For this review, use the dimensioned drawing (mm, ordinates from the lowest corner) and the shaded views. Coordinates: 2 decimals unless noted, no trailing zeros. Loops run counter-clockwise (first coordinate to the right, second up) from the corner with the lowest first, then second, coordinate; pieces in that order, holes last. Notation, with made-up numbers: M 2.25,53.25 L 6.25,53.25 A16 ccw 6.25,62.25 Z; hole C -26,9 d6. An arc over 180 degrees is marked long. Write item = value, one per line. Start each with the question number.
Q1. Mouldability with a two-part tool opening along X and no side actions: class the marked faces 1 and 2 as released by +X, released by -X, zero draft, split by the parting line, or undercut.
Q2. We need section A-A on z = 15.24. Give the boundary of the cut face in (x, y).
Q3. We need section B-B on x = 15.24. Give the boundary of the cut face in (y, z), and give its area (3 significant figures).
Q4. We need section D-D on y = 24. Give the boundary of the cut face in (x, z).
Q5. Wall thickness on probe 1 along X at (y, z) = (35.7, 15.24); probe 2 along X at (y, z) = (23.5, 15.24): over which ranges is each line inside the solid? List them lowest first.
Q6. Clearance check with flat-ended pins moving along their axes: pin 1 Ø10 at (x, y) = (26, 22) entering from -Z; pin 2 Ø5 at (y, z) = (29.5, 26.5) entering from +X; pin 3 Ø1.7 at (x, z) = (1.27, 15.24) entering from +Y. State where each tip first meets the part, or that it passes through.
Q7. We need section C-C on x = 1.27. Give the boundary of the cut face in (y, z).
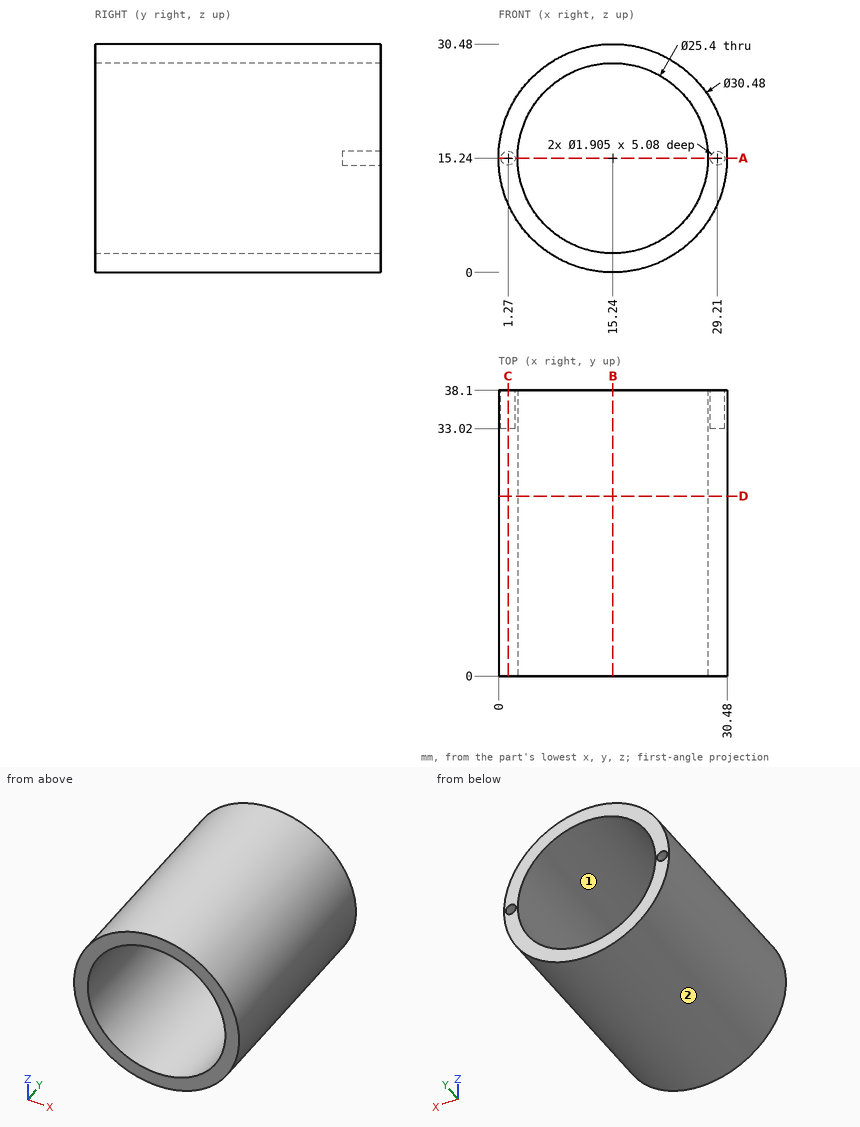
Returned:
q1.face_1 = undercut
q1.face_2 = split by the parting line
q2.outline = M 0,0 L 2.54,0 L 2.54,38.1 L 2.22,38.1 L 2.22,33.02 L 0.32,33.02 L 0.32,38.1 L 0,38.1 Z; M 27.94,0 L 30.48,0 L 30.48,38.1 L 30.16,38.1 L 30.16,33.02 L 28.26,33.02 L 28.26,38.1 L 27.94,38.1 Z
q3.outline = M 0,0 L 38.1,0 L 38.1,2.54 L 0,2.54 Z; M 0,27.94 L 38.1,27.94 L 38.1,30.48 L 0,30.48 Z
q3.area = 194 mm^2
q4.outline = C 15.24,15.24 d30.48; hole C 15.24,15.24 d25.4
q5.probe_1 = 0 to 0.32, 2.22 to 2.54, 27.94 to 28.26, 30.16 to 30.48
q5.probe_2 = 0 to 2.54, 27.94 to 30.48
q6.pin_1 = 1.13
q6.pin_2 = 27.71
q6.pin_3 = 33.02
q7.outline = M 0,9.15 L 38.1,9.15 L 38.1,14.29 L 33.02,14.29 L 33.02,16.19 L 38.1,16.19 L 38.1,21.33 L 0,21.33 Z
